from build123d import *

# Parameters (mm, degrees)
SKETCH_1_R      = 5.114284372
EXTRUDE_1_DEPTH = 10


with BuildPart() as part:
    # 草图1 → 凸台-拉伸1 (new body)
    with BuildSketch(Plane(origin=(0, 0, 0), x_dir=(1, 0, 0), z_dir=(0, 1, 0))):
        with BuildLine():
            Line((-83.772735406, 49.280387531), (-86.399180334, 44.731251472))
            Line((-86.399180334, 44.731251472), (-57.64544126, 26.631806208))
            ThreePointArc((-57.64544126, 26.631806208), (45.081659194, -44.720174467), (-27.095022974, 57.429171421))
            Line((-27.095022974, 57.429171421), (-38.463553205, 77.903659286))
            Line((-38.463553205, 77.903659286), (-42.624266956, 75.73666196))
            Line((-42.624266956, 75.73666196), (-47.35960117, 73.002715477))
            Line((-47.35960117, 73.002715477), (-35.578301324, 52.596905564))
            ThreePointArc((-35.578301324, 52.596905564), (-44.050696451, 45.736048607), (-51.224672516, 37.527095886))
            Line((-51.224672516, 37.527095886), (-80.420062365, 55.08738758))
            Line((-80.420062365, 55.08738758), (-83.772735406, 49.280387531))
        make_face()
        with Locations(Location((0, 0, 0), (0, 0, 270))):
            Circle(SKETCH_1_R, mode=Mode.SUBTRACT)
    extrude(amount=EXTRUDE_1_DEPTH)


solid = part.part
The model under review builds one solid part; all positions refer to its coordinate system, in mm. A direction names the side the tool comes from. Round coordinates to 2 decimals unless told otherwise and drop trailing zeros. Write each loop counter-clockwise with the first axis right and the second up, starting at its lowest first coordinate (ties: lowest second). Pieces come first, ordered by that corner, then holes. Notation, with made-up numbers: M 15.5,-31.5 L 23.5,-31.5 A21 ccw 23.5,-16.5 Z; hole C 42.5,4 d8. An arc over 180 degrees is marked long. Answer as CSV lines item,"result". Start each with the question number.
Q1. Consider section B-B, the plane x = 0. Give the boundary of the cut face in (y, z), then the cut area to 3 significant figures.
Q2. Tool access review of faces 4 (the face through (-72.224, 4.93, -35.808)), 5 (the face through (-43.94, 4.93, -45.84)), 6 (the face through (-65.618, 4.93, -46.184)): name each direction out of +Z, -Z, +X, -X, +Y, -Y from which nothing blocks a thin tool from reaching the whole face with its end or side.
Q3. Clearance check with flat-ended pins moving along their axes: P1, Ø3, axis at y = 5.5, z = -40, coming from the -X side; P2, Ø5, axis at x = -51, y = 6, coming from the +Z side. State where each tip first meets the part, or that it passes through.
Q4. Consider section A-A, the plane y = 8. Give the boundary of the cut face in (x, z), then the cut area to 3 significant figures.
Q5. The part is to be moulded in two halves that separate along Z. For faces 1 (the face through (-32.7, 4.93, -67.52)), 2 (the face through (5.07, 4.93, -0.67)), 3 (the face through (4, 10, -8)), say which applies: +Z half, -Z half, draft (parallel to the pull), parting line (faces both ways), or undercut.
Q6. Wall thickness on line 1 along X through (y, z) = (2.5, 0); line 2 along Z through (x, y) = (2.5, 1.5); line 3 along Z through (x, y) = (4, 3.25): over which ranges is each line inside the solid? List them lowest first.
Q7. Consider section C-C, the plane z = 0. Give the boundary of the cut face in (x, y).
Q8. Consider section D-D, the plane z = 40. Give the boundary of the cut face in (x, y).
Result set:
1,outline,"M 0,-63.5 L 10,-63.5 L 10,-5.11 L 0,-5.11 Z; M 0,5.11 L 10,5.11 L 10,63.5 L 0,63.5 Z"
1,area,"1,170 mm²"
2,face 4,"-X, +Y, -Y"
2,face 5,"+Y, -Y"
2,face 6,"-Z, +Y, -Y"
3,P1,"stops at x = -81.27"
3,P2,"stops at z = 40.99"
4,outline,"M -86.4,-44.73 L -80.42,-55.09 L -51.22,-37.53 A63.5 ccw -35.58,-52.6 L -47.36,-73 L -42.62,-75.74 L -38.46,-77.9 L -27.1,-57.43 A63.5 ccw long -57.65,-26.63 Z; hole C 0,0 d10.23"
4,area,"13,200 mm²"
5,face 1,"-Z half"
5,face 2,"undercut"
5,face 3,"draft"
6,line 1,"x = -63.5 to -5.11, 5.11 to 63.5"
6,line 2,"z = -63.45 to -4.46, 4.46 to 63.45"
6,line 3,"z = -63.37 to -3.19, 3.19 to 63.37"
7,outline,"M -63.5,0 L -5.11,0 L -5.11,10 L -63.5,10 Z; M 5.11,0 L 63.5,0 L 63.5,10 L 5.11,10 Z"
8,outline,"M -49.32,0 L 49.32,0 L 49.32,10 L -49.32,10 Z"
